CAD build for the part. Positions are in the model's coordinates, mm. Face numbers are marked on the shaded views. A direction names the side the tool comes from. Give positions to 0.01 mm unless a question says otherwise; leave off trailing zeros. Write each loop counter-clockwise with the first axis right and the second up, starting at its lowest first coordinate (ties: lowest second). Pieces come first, ordered by that corner, then holes. Notation, with made-up numbers: (44.25, 59.5) -> (55.25, 59.5) arc R15 ccw to (55.25, 63.5) -> close; hole circle Ø2 at (38.5, 9). An arc over 180 degrees is marked (long way). Use one line per item in the form item = value. Start each with the question number.
Solid Edge part; units mm, degrees
sketch "Sketch1" plane through (0, 0, 0) normal (0, -1, 0) x (1, 0, 0)
  line L0 (47, 70.8) -> (35, 70.8)
  line L1 (35, 70.8) -> (35, 85.8)
  line L2 (28, 85.8) -> (35, 85.8)
  line L3 (28, 76.8) -> (28, 85.8)
  line L4 (31, 76.8) -> (28, 76.8)
  line L5 (31, 0) -> (31, 76.8)
  line L6 (31, 0) -> (47, 0)
  line L7 (47, 0) -> (47, 11)
  line L8 (47, 11) -> (35, 11)
  line L9 (35, 11) -> (35, 60.8)
  line L10 (35, 60.8) -> (47, 60.8)
  line L11 (47, 60.8) -> (47, 70.8)
revolve "RevolvedProtrusion1" add sketch "Sketch1" angle 360 about axis through (0, 0, 0) along (0, 0, 1)
hole "Hole1" at (-41, 0, 70.8) direction (0, 0, -1) diameter 6.5 end up to next
pattern_circular "Pattern1" count 8 over 360 about axis through (0, 0, 70.8) along (0, 0, -1) of "Hole1"
hole "Agujero_3" at (-41, 0, 0) direction (0, 0, 1) diameter 4.917 end through all
pattern_circular "Pattern3" count 8 over 360 about axis through (0, 0, 0) along (0, 0, 1) of "Agujero_3"
properties part number "1976-1100-006" material "Aluminio, 7075-T6"
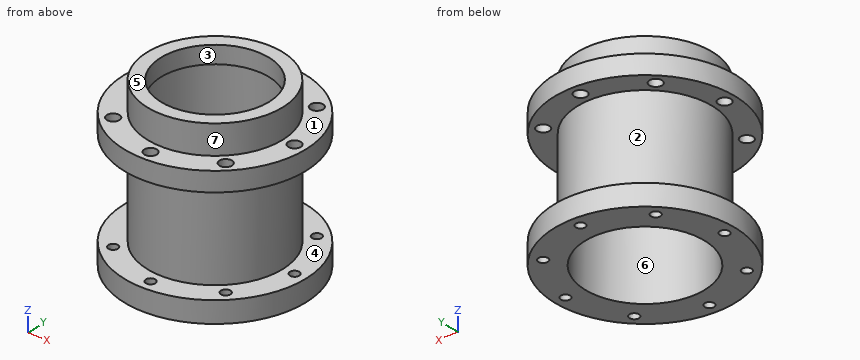
1) Cut at C-C (x = 41). Give the cut face in (y, z).
2) Wall check: line 1 along Y through (x, z) = (0, 65); line 2 along Z through (x, y) = (-42.5, -9); line 3 along X through (y, z) = (1, 41.5). Give the ranges that are in metal, low to high. Write a range as from..to.
3) Cut at B-B (x = -10.5). Give the cut face in (y, z), and give its area (3 significant figures).
4) Pin check, flat tips, straight feed: pin 1 (1 mm diameter, centred on x = 31.5, y = 33.5, fed in from +Z); pin 2 (4 mm diameter, centred on y = 31.5, z = 32, fed in from +X); pin 3 (8 mm diameter, centred on x = -41, y = 0, fed in from -Z); pin 4 (10 mm diameter, centred on x = -19.5, z = 48, fed in from -Y). Stop position of each tip, or through.
5) Two-plate mould, pull along Z, no slides. Class the marked faces 1, 2 and 3: released by +Z, released by -Z, zero draft, split by the parting line, or undercut.
6) Cut at A-A (y = -7). Give the cut face in (x, z), and give its area (3 significant figures).
7) 3-axis set-ups, long thin cutter, end or side, ignore diameter. For the marked faces 4, 5, 6 and 7: which of +Z, -Z, +X, -X, +Y, -Y reach the whole face in a straight line?
Final values:
q1.outline = (-22.98, 0) -> (-2.46, 0) -> (-2.46, 11) -> (-22.98, 11) -> close; (-22.98, 60.8) -> (-3.25, 60.8) -> (-3.25, 70.8) -> (-22.98, 70.8) -> close; (2.46, 0) -> (22.98, 0) -> (22.98, 11) -> (2.46, 11) -> close; (3.25, 60.8) -> (22.98, 60.8) -> (22.98, 70.8) -> (3.25, 70.8) -> close
q2.line_1 = -47..-44.25, -37.75..-31, 31..37.75, 44.25..47
q2.line_2 = 0..11, 60.8..70.8
q2.line_3 = -34.99..-30.98, 30.98..34.99
q3.outline = (-45.81, 0) -> (-29.17, 0) -> (-29.17, 76.8) -> (-25.96, 76.8) -> (-25.96, 85.8) -> (-33.39, 85.8) -> (-33.39, 70.8) -> (-45.81, 70.8) -> (-45.81, 60.8) -> (-33.39, 60.8) -> (-33.39, 11) -> (-45.81, 11) -> close; (25.96, 76.8) -> (29.17, 76.8) -> (29.17, 0) -> (45.81, 0) -> (45.81, 11) -> (33.39, 11) -> (33.39, 60.8) -> (45.81, 60.8) -> (45.81, 70.8) -> (33.39, 70.8) -> (33.39, 85.8) -> (25.96, 85.8) -> close
q3.area = 1,300 mm^2
q4.pin_1 = 70.8
q4.pin_2 = 18.83
q4.pin_3 = 0
q4.pin_4 = -31.86
q5.face_1 = released by +Z
q5.face_2 = undercut
q5.face_3 = zero draft
q6.outline = (-46.48, 0) -> (-30.2, 0) -> (-30.2, 76.8) -> (-27.11, 76.8) -> (-27.11, 85.8) -> (-34.29, 85.8) -> (-34.29, 70.8) -> (-46.48, 70.8) -> (-46.48, 60.8) -> (-34.29, 60.8) -> (-34.29, 11) -> (-46.48, 11) -> close; (27.11, 76.8) -> (30.2, 76.8) -> (30.2, 0) -> (46.48, 0) -> (46.48, 11) -> (34.29, 11) -> (34.29, 60.8) -> (46.48, 60.8) -> (46.48, 70.8) -> (34.29, 70.8) -> (34.29, 85.8) -> (27.11, 85.8) -> close
q6.area = 1,270 mm^2
q7.face_4 = none
q7.face_5 = +Z, +X, -X, +Y, -Y
q7.face_6 = -Z
q7.face_7 = +Z
